Geometry check sheet. Reference: the model listing, model coordinates, mm. A direction names the side the tool comes from. Give positions to 0.01 mm unless a question says otherwise; leave off trailing zeros. Write each loop counter-clockwise with the first axis right and the second up, starting at its lowest first coordinate (ties: lowest second). Pieces come first, ordered by that corner, then holes. Notation, with made-up numbers: (48.5, -23) - (73.5, -23) arc R20 cw to (73.5, 16) - close; hole circle Ø8 at (20.5, -33.5). An arc over 180 degrees is marked (long way). Use a Markdown table: item, result.
```python
from build123d import *

# Parameters (mm, degrees)
RESSALTO_EXTRUS_O1_DEPTH = 11
ESBO_O2_W                = 10
ESBO_O2_H                = 1.5
RESSALTO_EXTRUS_O2_DEPTH = 7
RESSALTO_EXTRUS_O3_DEPTH = 2
ESBO_O4_R                = 1.55
CORTE_EXTRUS_O1_DEPTH    = 2
CORTE_EXTRUS_O2_DEPTH    = 37.687872656


with BuildPart() as part:
    # Esboço1 → Ressalto-extrusão1 (new body)
    with BuildSketch(Plane.XY):
        with BuildLine():
            Line((-5, -5), (0, -5))
            ThreePointArc((0, -5), (-3.535533906, -3.535533906), (-5, 0))
            Line((-5, 0), (-5, -5))
        make_face()
        with BuildLine():
            Line((5, -5), (5, 0))
            ThreePointArc((5, 0), (3.535533906, -3.535533906), (0, -5))
            Line((0, -5), (5, -5))
        make_face()
        with BuildLine():
            ThreePointArc((-3.5, 0), (0, 3.5), (3.5, 0))
            Line((3.5, 0), (5, 0))
            ThreePointArc((5, 0), (3.535533906, 3.535533905), (1e-09, 5))
            ThreePointArc((1e-09, 5), (-3.535533905, 3.535533906), (-5, 0))
            Line((-5, 0), (-3.5, 0))
        make_face()
        with BuildLine():
            Line((5, 0), (3.5, 0))
            ThreePointArc((3.5, 0), (0, -3.5), (-3.5, 0))
            Line((-3.5, 0), (-5, 0))
            ThreePointArc((-5, 0), (-3.535533906, -3.535533906), (0, -5))
            ThreePointArc((0, -5), (3.535533906, -3.535533906), (5, 0))
        make_face()
    ressalto_extrus_o1 = extrude(amount=RESSALTO_EXTRUS_O1_DEPTH)

    # Esboço2 → Ressalto-extrusão2 (add)
    with BuildSketch(Plane.XY.offset(11)):
        with Locations((0, -4.25)):
            Rectangle(ESBO_O2_W, ESBO_O2_H)
    ressalto_extrus_o2 = extrude(amount=RESSALTO_EXTRUS_O2_DEPTH)

    # Esboço3 → Ressalto-extrusão3 (add)
    with BuildSketch(Plane.XY.offset(18)):
        with BuildLine():
            Line((3.5, -3.5), (5, -3.5))
            ThreePointArc((5, -3.5), (4.25, -2.75), (3.5, -3.5))
        make_face()
        with BuildLine():
            Line((-5, -3.5), (-3.5, -3.5))
            ThreePointArc((-3.5, -3.5), (-4.25, -2.75), (-5, -3.5))
        make_face()
    ressalto_extrus_o3 = extrude(amount=-RESSALTO_EXTRUS_O3_DEPTH)

    # Espelhar1: Ressalto-extrusão1, Ressalto-extrusão2, Ressalto-extrusão3 across plane
    add(ressalto_extrus_o1.mirror(Plane(origin=(0, 0, 18), x_dir=(1, 0, 0), z_dir=(0, 0, -1))))
    add(ressalto_extrus_o2.mirror(Plane(origin=(0, 0, 18), x_dir=(1, 0, 0), z_dir=(0, 0, -1))))
    add(ressalto_extrus_o3.mirror(Plane(origin=(0, 0, 18), x_dir=(1, 0, 0), z_dir=(0, 0, -1))))

    # Esboço4 → Corte-extrusão1 (cut)
    with BuildSketch(Plane(origin=(0, -3.5, 0), x_dir=(1, 0, 0), z_dir=(0, 1, 0))):
        with Locations(Location((0, -18, 0), (0, 0, 270))):
            Circle(ESBO_O4_R)
    extrude(amount=-CORTE_EXTRUS_O1_DEPTH, mode=Mode.SUBTRACT)

    # Esboço5 → Corte-extrusão2 (cut, through all)
    with BuildSketch(Plane.XY.offset(36)):
        with BuildLine():
            Line((2.449489743, -2.5), (5, -2.5))
            Line((5, -2.5), (5, 0))
            ThreePointArc((5, 0), (4.766431527, 1.510341187), (4.087547799, 2.87957514))
            Line((4.087547799, 2.87957514), (2.861283459, 2.015702598))
            ThreePointArc((2.861283459, 2.015702598), (3.336502069, 1.057238831), (3.5, 0))
            ThreePointArc((3.5, 0), (3.226702194, -1.355873501), (2.449489743, -2.5))
        make_face()
    extrude(amount=-CORTE_EXTRUS_O2_DEPTH, mode=Mode.SUBTRACT)


solid = part.part
```
1) Section check B-B on y = -2. Record the boundary of the cut face in (x, z).
Working result:
| item | result |
|---|---|
| outline | (-5, 0) - (-2.87, 0) - (-2.87, 11) - (-5, 11) - close; (-5, 25) - (-2.87, 25) - (-2.87, 36) - (-5, 36) - close |
2) Section check A-A on z = 18. Record the boundary of the cut face in (x, y), then the cut area to 3 significant figures.
Working result:
| item | result |
|---|---|
| outline | (-5, -5) - (-1.55, -5) - (-1.55, -3.5) - (-3.5, -3.5) arc R0.75 ccw to (-5, -3.5) - close; (1.55, -5) - (5, -5) - (5, -3.5) arc R0.75 ccw to (3.5, -3.5) - (1.55, -3.5) - close |
| area | 12.1 mm² |
3) Material ranges on L1, parallel to Z at x = -4.5, y = 2; L2, parallel to Y at x = 4.5, z = 22; L3, parallel to Y at x = 2.25, z = 34.5, recorded low to high. Write a range as from..to.
Working result:
| item | result |
|---|---|
| L1 | z = 0..11, 25..36 |
| L2 | y = -5..-3.5 |
| L3 | y = -5..-2.68, 2.68..4.47 |
4) Set-up check for faces 5 (the flat face through (3, -3, 11)), 6 (the flat face through (0, -3.5, 20)), 7 (the flat face through (4, -2.5, 31)): record each of +Z, -Z, +X, -X, +Y, -Y from which the full face is reachable in a straight line by a thin tool's end or side.
Working result:
| item | result |
|---|---|
| face 5 | +X, -X, +Y |
| face 6 | +Y |
| face 7 | +Z, -Z, +X |
5) Section check C-C on z = 30. Record the boundary of the cut face in (x, y).
Working result:
| item | result |
|---|---|
| outline | (-5, -5) - (5, -5) - (5, -2.5) - (2.45, -2.5) arc R3.5 cw (long way) to (2.86, 2.02) - (4.09, 2.88) arc R5 ccw to (-5, 0) - close |
6) Section check D-D on x = -4. Record the boundary of the cut face in (y, z).
Working result:
| item | result |
|---|---|
| outline | (-5, 0) - (3, 0) - (3, 11) - (-3.5, 11) - (-3.5, 16) - (-2.79, 16) - (-2.79, 20) - (-3.5, 20) - (-3.5, 25) - (3, 25) - (3, 36) - (-5, 36) - close |
7) Depth check by flat-ended pin: P1, Ø5, axis at y = -1.5, z = 30, coming from the +X side; P2, Ø2, axis at x = 4, z = 31.5, coming from the +Y side. Enter the tip coordinate at first touch or a pass-through.
Working result:
| item | result |
|---|---|
| P1 | stops at x = 5 |
| P2 | stops at y = 4 |
8) Mould release check, pull along Z, two halves, no side actions. Record for faces 1 (the flat face through (-3.4, -2.2, 0)), 2 (the flat face through (-3.4, -2.2, 36)), 3 (the flat face through (4, -2.5, 6)), 4 (the cylindrical face through (4.27, -2.75, 17.97)): pulls with the +Z half, pulls with the -Z half, needs draft (parallel to the pull), parting line crosses it, or undercut.
Working result:
| item | result |
|---|---|
| face 1 | pulls with the -Z half |
| face 2 | pulls with the +Z half |
| face 3 | needs draft |
| face 4 | undercut |
